For this review, take the finished solid that the model builds, in its own axes (mm). A direction names the side the tool comes from. Coordinates: 2 decimals unless noted, no trailing zeros. Write each loop counter-clockwise with the first axis right and the second up, starting at its lowest first coordinate (ties: lowest second). Pieces come first, ordered by that corner, then holes.
```python
from build123d import *

# Parameters (mm, degrees)
SKETCH1_R           = 21
BOSS_EXTRUDE1_DEPTH = 7
SKETCH2_R           = 30
BOSS_EXTRUDE2_DEPTH = 3
SKETCH3_R           = 16
CUT_EXTRUDE1_DEPTH  = 44.588989435
SKETCH4_R           = 1.5
CUT_EXTRUDE2_DEPTH  = 5
BOSS_EXTRUDE3_START = -3
SKETCH5_R           = 16
SKETCH5_R_2         = 15
BOSS_EXTRUDE3_DEPTH = 3
SKETCH6_R           = 2
CUT_EXTRUDE3_DEPTH  = 44


with BuildPart() as part:
    # Sketch1 → Boss-Extrude1 (new body)
    with BuildSketch(Plane(origin=(0, 0, 0), x_dir=(0, 0, -1), z_dir=(1, 0, 0))):
        Circle(SKETCH1_R)
    extrude(amount=BOSS_EXTRUDE1_DEPTH)

    # Sketch2 → Boss-Extrude2 (add)
    with BuildSketch(Plane(origin=(7, 0, 0), x_dir=(0, 0, -1), z_dir=(1, 0, 0))):
        Circle(SKETCH2_R)
    extrude(amount=BOSS_EXTRUDE2_DEPTH)

    # Sketch3 → Cut-Extrude1 (cut, through all)
    with BuildSketch(Plane.ZY):
        Circle(SKETCH3_R)
    extrude(amount=-CUT_EXTRUDE1_DEPTH, mode=Mode.SUBTRACT)

    # Sketch4 → Cut-Extrude2 (cut)
    with BuildSketch(Plane.ZY):
        with Locations((0, 18.5)):
            Circle(SKETCH4_R)
        with Locations((18.5, 0)):
            Circle(SKETCH4_R)
        with Locations((0, -18.5)):
            Circle(SKETCH4_R)
        with Locations((-18.5, 0)):
            Circle(SKETCH4_R)
    extrude(amount=-CUT_EXTRUDE2_DEPTH, mode=Mode.SUBTRACT)

    # Sketch5 → Boss-Extrude3 (add)
    with BuildSketch(Plane(origin=(10, 0, 0), x_dir=(0, 0, -1), z_dir=(1, 0, 0)).offset(BOSS_EXTRUDE3_START)):
        with Locations(Location((0, 0, 0), (0, 0, 180))):
            Circle(SKETCH5_R)
        Circle(SKETCH5_R_2, mode=Mode.SUBTRACT)
    extrude(amount=BOSS_EXTRUDE3_DEPTH)

    # Sketch6 → Cut-Extrude3 (cut, through all)
    with BuildSketch(Plane.ZY.offset(-7)):
        with Locations((0, 26)):
            Circle(SKETCH6_R)
        with Locations((26, 0)):
            Circle(SKETCH6_R)
        with Locations((0, -26)):
            Circle(SKETCH6_R)
        with Locations((-26, 0)):
            Circle(SKETCH6_R)
    extrude(amount=-CUT_EXTRUDE3_DEPTH, mode=Mode.SUBTRACT)


solid = part.part
```
Q1. For probe 1 along Y at (x, z) = (3.25, 0); probe 2 along Y at (x, z) = (7.9, 0); probe 3 along X at (y, z) = (-17.5, 20), list the stretches that pass through material, from the lowest coordinate up.
Ans:
probe 1: y = -21 to -20, -17 to -16, 16 to 17, 20 to 21
probe 2: y = -30 to -28, -24 to -15, 15 to 24, 28 to 30
probe 3: x = 7 to 10
Q2. Add section C-C (z = 9). State the section outline as (x, y) points, then the cut area to 3 significant figures.
Ans:
outline: (0, -18.97) - (7, -18.97) - (7, -28.62) - (10, -28.62) - (10, -12) - (7, -12) - (7, -13.23) - (0, -13.23) - close; (0, 13.23) - (7, 13.23) - (7, 12) - (10, 12) - (10, 28.62) - (7, 28.62) - (7, 18.97) - (0, 18.97) - close
area: 180 mm2
Q3. Clearance check with flat-ended pins moving along their axes: pin 1 Ø6 at (x, y) = (7.5, 18.5) entering from +Z; pin 2 Ø1.5 at (x, y) = (6.5, -2) entering from -Z; pin 3 Ø3 at (x, y) = (4.5, -3) entering from -Z; pin 4 Ø3 at (y, z) = (0, 26) entering from +X. State where each tip first meets the part, or that it passes through.
Ans:
pin 1: stops at z = 25.69
pin 2: stops at z = -29.97
pin 3: stops at z = -20.95
pin 4: passes through
Q4. Add section D-D (x = 8.5). State the section outline as (y, z) points.
Ans:
outline: circle Ø60 at (0, 0); hole circle Ø4 at (-26, 0); hole circle Ø30 at (0, 0); hole circle Ø4 at (0, -26); hole circle Ø4 at (0, 26); hole circle Ø4 at (26, 0)
Q5. Add section B-B (z = 0). Give the number of separate pieces and of enclosed holes in the cut face, then the cut area to 3 significant figures.
Ans:
separate pieces: 4
enclosed holes: 0
area: 106 mm2
Q6. Draft analysis for pull direction Y (two halves, no side actions). For faces 1 (the cylindrical face through (3.45, 6.31, -20.03)), 2 (the flat face through (7, 17.9, 11.3)), 3 (the flat face through (5, 0, -19)), state which applies: +Y half, -Y half, draft (parallel to the pull), parting line (faces both ways), or undercut.
Ans:
face 1: parting line
face 2: draft
face 3: undercut
Q7. Add section A-A (y = 11). State the section outline as (x, z) points, then the cut area to 3 significant figures.
Ans:
outline: (0, -17.89) - (7, -17.89) - (7, -27.91) - (10, -27.91) - (10, -10.2) - (7, -10.2) - (7, -11.62) - (0, -11.62) - close; (0, 11.62) - (7, 11.62) - (7, 10.2) - (10, 10.2) - (10, 27.91) - (7, 27.91) - (7, 17.89) - (0, 17.89) - close
area: 194 mm2
Q8. Tool access review of faces 4 (the cylindrical face through (2, 0, 17)), 5 (the cylindrical face through (8.479, 0.66, 14.985)): name each direction out of +Z, -Z, +X, -X, +Y, -Y from which nothing blocks a thin tool from reaching the whole face with its end or side.
Ans:
face 4: -X
face 5: +X, -X
